The figure shows three views and two pictorial views of one solid part (mm, origin at its lowest corner). Answer the questions. A direction names the side the tool comes from. Round coordinates to 2 decimals unless told otherwise and drop trailing zeros. Order: outer loops, then holes, each group sorted by start corner. A loop starts at its lowest first (then second) coordinate and runs counter-clockwise, first axis right, second up. Notation, with made-up numbers: (20, -36) -> (48, -36) arc R16 cw to (48, -20) -> close; hole circle Ø3 at (-6.5, 21.5). An arc over 180 degrees is marked (long way). Answer in a Markdown table with one row per item. Add a question column.
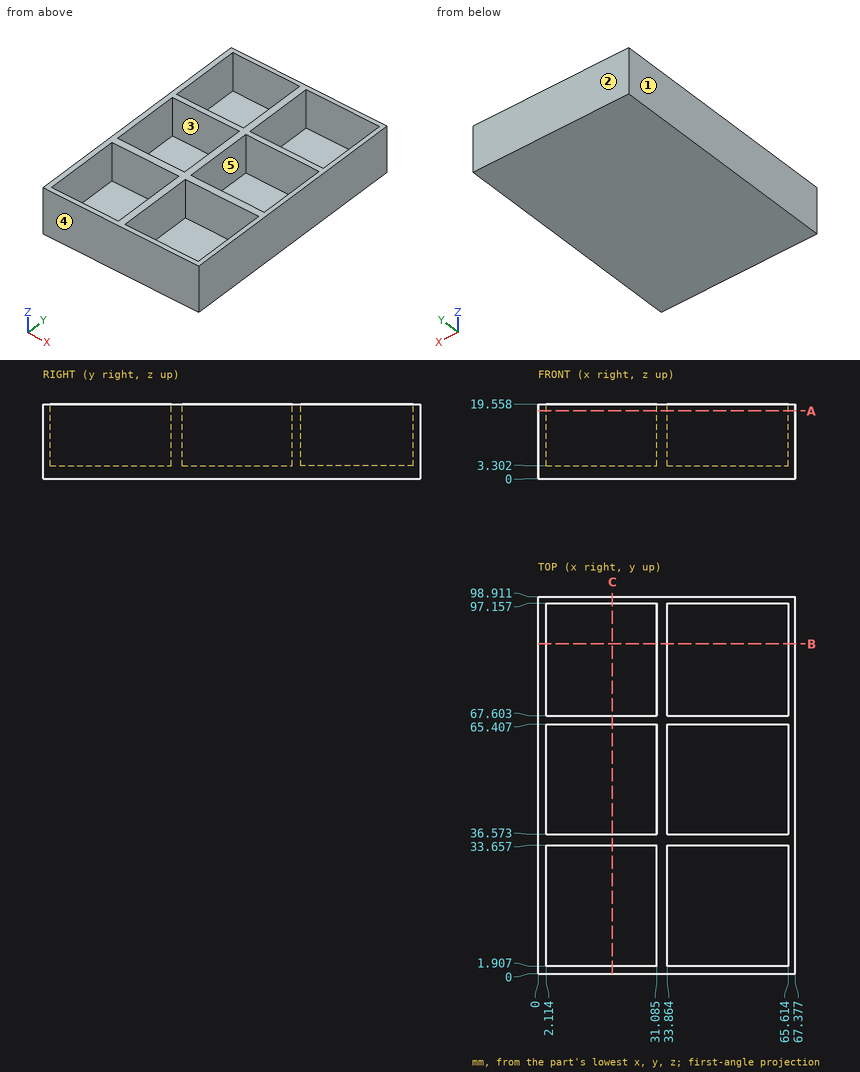
1. The part is cut by section C-C (x = 19.5). Give the vertices of the cut face in (y, z).
2. The mould has two halves that part along X. Classify the marked faces 1, 2 and 3: released by +X, released by -X, zero draft, split by the parting line, or undercut.
3. For the marked faces 4 and 5, determine the directions among +Z, -Z, +X, -X, +Y, -Y from which every point of the face is accessible in a straight line to the end or side of a thin tool.
4. The part is cut by section B-B (y = 86.5). Give the vertices of the cut face in (x, z) (1 decimal).
5. Straight lines are drawn through the part: line 1 along X through (y, z) = (16, 9) (1 decimal); line 2 along Y through (x, z) = (36.5, 16); line 3 along Z through (x, y) = (44.5, 50). For each, find the intervals that lie inside material, in ascending order.
6. This flat-tipped pin is pushed along its axis until it touches: pin 1 (8.5 mm diameter, centred on x = 57.5, y = 49.5, fed in from +Z). Where does it stop, or does it pass through?
7. The part is cut by section A-A (z = 17.75). Give the vertices of the cut face in (x, y) (1 decimal), then the cut area to 3 significant figures.
Report:
| question | item | result |
|---|---|---|
| 1 | outline | (0, 0) -> (98.91, 0) -> (98.91, 19.56) -> (97.16, 19.56) -> (97.16, 3.3) -> (67.6, 3.3) -> (67.6, 19.56) -> (65.41, 19.56) -> (65.41, 3.3) -> (36.57, 3.3) -> (36.57, 19.56) -> (33.66, 19.56) -> (33.66, 3.3) -> (1.91, 3.3) -> (1.91, 19.56) -> (0, 19.56) -> close |
| 2 | face 1 | released by -X |
| 2 | face 2 | zero draft |
| 2 | face 3 | undercut |
| 3 | face 4 | +Z, -Z, +X, -X, -Y |
| 3 | face 5 | +Z |
| 4 | outline | (0, 0) -> (67.4, 0) -> (67.4, 19.6) -> (65.6, 19.6) -> (65.6, 3.3) -> (33.9, 3.3) -> (33.9, 19.6) -> (31.1, 19.6) -> (31.1, 3.3) -> (2.1, 3.3) -> (2.1, 19.6) -> (0, 19.6) -> close |
| 5 | line 1 | x = 0 to 2.1, 31.1 to 33.9, 65.6 to 67.4 |
| 5 | line 2 | y = 0 to 1.91, 33.66 to 36.57, 65.41 to 67.6, 97.16 to 98.91 |
| 5 | line 3 | z = 0 to 3.3 |
| 6 | pin 1 | stops at z = 3.3 |
| 7 | outline | (0, 0) -> (67.4, 0) -> (67.4, 98.9) -> (0, 98.9) -> close; hole (2.1, 1.9) -> (31.1, 1.9) -> (31.1, 33.7) -> (2.1, 33.7) -> close; hole (2.1, 36.6) -> (31.1, 36.6) -> (31.1, 65.4) -> (2.1, 65.4) -> close; hole (2.1, 67.6) -> (31.1, 67.6) -> (31.1, 97.2) -> (2.1, 97.2) -> close; hole (33.9, 1.9) -> (65.6, 1.9) -> (65.6, 33.7) -> (33.9, 33.7) -> close; hole (33.9, 36.6) -> (65.6, 36.6) -> (65.6, 65.4) -> (33.9, 65.4) -> close; hole (33.9, 67.6) -> (65.6, 67.6) -> (65.6, 97.2) -> (33.9, 97.2) -> close |
| 7 | area | 1,190 mm^2 |
